from build123d import *

# Parameters (mm, degrees)
F0_W     = 152.4
F0_H     = 50.8
F1_DEPTH = 25.4
F3_W     = 338.114095
F3_H     = 181.983536
F3_W_2   = 314.57949
F3_H_2   = 152.960297
F4_DEPTH = 6.35
F2_R     = 16.51
F5_DEPTH = 25.4


with BuildPart() as f1:
    # F0 (on Top) → F1 (new body)
    with BuildSketch(Plane.XY):
        Polygon((0, 76.2), (0, 0), (355.6, 0), (355.6, 203.2), (0, 203.2), (0, 127), align=None)
        with Locations((-76.2, 101.6)):
            Rectangle(F0_W, F0_H)
    extrude(amount=F1_DEPTH)

    # F3 (on face) → F4 (join)
    with BuildSketch(Plane.XY.offset(25.4)):
        with Locations((178.495669, 98.406327)):
            Rectangle(F3_W, F3_H)
        with Locations((177.711187, 98.79853)):
            Rectangle(F3_W_2, F3_H_2, mode=Mode.SUBTRACT)
    extrude(amount=F4_DEPTH)

    # F2 (on face) → F5 (cut)
    with BuildSketch(Plane.XY.offset(25.4)):
        with Locations((-123.133972, 101.54397)):
            Circle(F2_R)
    extrude(amount=-F5_DEPTH, mode=Mode.SUBTRACT)


solid = f1.part
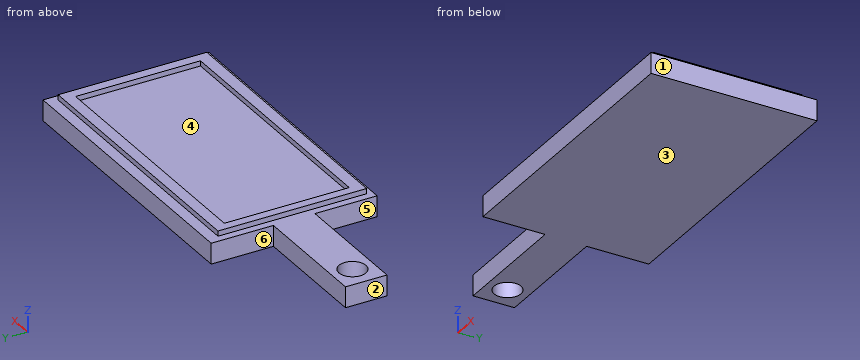
The model under review builds one solid part; all positions refer to its coordinate system, in mm. Face numbers are marked on the shaded views. A direction names the side the tool comes from. Give positions to 0.01 mm unless a question says otherwise; leave off trailing zeros. Loops run counter-clockwise (first coordinate to the right, second up) from the corner with the lowest first, then second, coordinate; pieces in that order, holes last. Notation, with made-up numbers: (49.25, -33.5) -> (101.25, -33.5) arc R16 ccw to (101.25, -25.5) -> close; hole circle Ø6 at (19, -15). An arc over 180 degrees is marked (long way). Answer as a JSON object with one key per item and string values. Group by question number.
Q1. Insertion check: pin 1 (1.9 mm diameter, centred on x = 100.5, z = 29.5, fed in from -Y); pin 2 (1 mm diameter, centred on x = 170.5, y = 60.5, fed in from +Z); pin 3 (7.5 mm diameter, centred on x = -66.5, z = 12.5, fed in from +Y). Each pin has a flat end and moves straight along its axis. Give the tip position at first contact, or say it passes through.
Q2. Take a section at C-C (y = 94.5). Write out the cut boundary in (x, z).
Q3. Draft analysis for pull direction X (two halves, no side actions). For the marked faces 1, 2, 3 and 4, state which applies: pulls with the +X half, pulls with the -X half, needs draft (parallel to the pull), parting line crosses it, or undercut.
Q4. Take a section at B-B (z = 13). Write out the cut boundary in (x, y), plus the area to 3 significant figures.
Q5. Tool access review of the marked faces 5 and 6: name each direction out of +Z, -Z, +X, -X, +Y, -Y from which nothing blocks a thin tool from reaching the whole face with its end or side.
Q6. Wall thickness on line 1 along Y through (x, z) = (22, 30.5); line 2 along Z through (x, y) = (117, 82); line 3 along Y through (x, z) = (-97, 15): over which ranges is each line inside the solid? List them lowest first.
Q7. Take a section at A-A (y = 63). Write out the cut boundary in (x, z), plus the area to 3 significant figures.
Q8. Take a section at D-D (x = 144). Write out the cut boundary in (y, z), plus the area to 3 significant figures.
Answer below:
{
 "1": {"pin 1": "stops at y = 7.41", "pin 2": "stops at z = 25.4", "pin 3": "stops at y = 127"},
 "2": {"outline": "(-152.4, 0) -> (-138.07, 0) -> (-138.07, 25.4) -> (-152.4, 25.4) -> close; (-108.2, 0) -> (355.6, 0) -> (355.6, 25.4) -> (347.55, 25.4) -> (347.55, 31.75) -> (335, 31.75) -> (335, 25.4) -> (20.42, 25.4) -> (20.42, 31.75) -> (9.44, 31.75) -> (9.44, 25.4) -> (-108.2, 25.4) -> close"},
 "3": {"face 1": "pulls with the +X half", "face 2": "pulls with the -X half", "face 3": "needs draft", "face 4": "undercut"},
 "4": {"outline": "(-152.4, 76.2) -> (0, 76.2) -> (0, 0) -> (355.6, 0) -> (355.6, 203.2) -> (0, 203.2) -> (0, 127) -> (-152.4, 127) -> close; hole circle Ø33.02 at (-123.13, 101.54)", "area": "79,100 mm2"},
 "5": {"face 5": "+Z, -Z, -X, -Y", "face 6": "+Z, -Z, -X, +Y"},
 "6": {"line 1": "y = 7.41 to 22.32, 175.28 to 189.4", "line 2": "z = 0 to 25.4", "line 3": "y = 76.2 to 127"},
 "7": {"outline": "(0, 0) -> (355.6, 0) -> (355.6, 25.4) -> (347.55, 25.4) -> (347.55, 31.75) -> (335, 31.75) -> (335, 25.4) -> (20.42, 25.4) -> (20.42, 31.75) -> (9.44, 31.75) -> (9.44, 25.4) -> (0, 25.4) -> close", "area": "9,180 mm2"},
 "8": {"outline": "(0, 0) -> (203.2, 0) -> (203.2, 25.4) -> (189.4, 25.4) -> (189.4, 31.75) -> (175.28, 31.75) -> (175.28, 25.4) -> (22.32, 25.4) -> (22.32, 31.75) -> (7.41, 31.75) -> (7.41, 25.4) -> (0, 25.4) -> close", "area": "5,350 mm2"}
}
